The listing builds one solid part. Answer for the finished solid, in the listing's coordinates (mm). A direction names the side the tool comes from. Give positions to 0.01 mm unless a question says otherwise; leave off trailing zeros. Order: outer loops, then holes, each group sorted by start corner. A loop starts at its lowest first (then second) coordinate and runs counter-clockwise, first axis right, second up. Notation, with made-up numbers: (82.25, 22.25) -> (127.25, 22.25) arc R22 cw to (127.25, 39.25) -> close; hole circle Ø9 at (3, 20.5). An arc over 180 degrees is marked (long way). One line per question, with ' | ' between items. Start each with the question number.
```python
from build123d import *

# Parameters (mm, degrees)
SKETCH_2_W          = 2
SKETCH_2_H          = 4.593987872
SKETCH_2_H_2        = 6.667892238
CUT_EXTRUDE_1_DEPTH = 39.5


with BuildPart() as part:
    # 草图1 → 旋转1 (revolve)
    with BuildSketch(Plane.XY, mode=Mode.PRIVATE) as revolve_1_sk:
        Polygon((-23.5, 11), (-26, 11), (-26, 7), (-25.5, 7), (-25.5, 6), (-28, 6), (-28, 5), (-25.5, 5), (-25.5, 4), (-26, 4), (-26, 0), (-23.5, 0), align=None)
    revolve(revolve_1_sk.sketch.rotate(Axis((0, 22.677499451, 0), (0, -1, 0)), 270), axis=Axis((0, 22.677499451, 0), (0, -1, 0)))  # turned: the seam where the file's is

    # 草图2 → 切除-拉伸1 (cut, symmetric)
    with BuildSketch(Plane(origin=(0, 0, 0), x_dir=(0, 0, -1), z_dir=(1, 0, 0))):
        with Locations((0, 11.296993936)):
            Rectangle(SKETCH_2_W, SKETCH_2_H)
        with Locations((0, -1.333946119)):
            Rectangle(SKETCH_2_W, SKETCH_2_H_2)
    extrude(amount=CUT_EXTRUDE_1_DEPTH, both=True, mode=Mode.SUBTRACT)


solid = part.part
```
(1) Determine the mould class of faces 5 (the face through (24.9, 4.5, -5.5)), 6 (the face through (-6, 5, 25)), 7 (the face through (-25, 2, 0)) for opening direction Z: pulls with the +Z half, pulls with the -Z half, needs draft (parallel to the pull), parting line crosses it, or undercut.
(2) The part is cut by section B-B on x = 0. Determine the outline of the cut face in (y, z).
(3) Consider line 1 (Y direction, x = 25.5, z = -4.5); line 2 (X direction, y = 3.5, z = 0); line 3 (Z direction, x = -3.5, y = 6.25). Determine where each line is inside the solid, lowest interval first.
(4) The part is cut by section A-A on z = 0. Determine the outline of the cut face in (x, y).
(5) Given P1, Ø6, axis at y = 9.5, z = -17, coming from the -X side; P2, Ø1.6, axis at x = -25, z = 0, coming from the -Y side; P3, Ø5, axis at y = 9, z = 3.5, coming from the -X side, each flat-ended and moving along its own axis, determine where each tip first touches the part or whether it passes through.
(6) For faces 1 (the face through (15.821, 8.972, -20.633)), 2 (the face through (19.1, 7, 17.2)), 3 (the face through (-25, 10, 1)), 4 (the face through (25, 2, 0)), determine the directions among +Z, -Z, +X, -X, +Y, -Y from which every point of the face is accessible in a straight line to the end or side of a thin tool.
Result sheet:
1) face 5: parting line crosses it | face 6: needs draft | face 7: undercut
2) outline: (0, -26) -> (4, -26) -> (4, -25.5) -> (5, -25.5) -> (5, -28) -> (6, -28) -> (6, -25.5) -> (7, -25.5) -> (7, -26) -> (11, -26) -> (11, -23.5) -> (0, -23.5) -> close; (0, 23.5) -> (11, 23.5) -> (11, 26) -> (7, 26) -> (7, 25.5) -> (6, 25.5) -> (6, 28) -> (5, 28) -> (5, 25.5) -> (4, 25.5) -> (4, 26) -> (0, 26) -> close
3) line 1: y = 0 to 4, 5 to 6, 7 to 11 | line 2: x = -26 to -23.5, 23.5 to 26 | line 3: z = -25.26 to -23.24, 23.24 to 25.26
4) outline: (-28, 5) -> (-25.5, 5) -> (-25.5, 4) -> (-26, 4) -> (-26, 2) -> (-23.5, 2) -> (-23.5, 9) -> (-26, 9) -> (-26, 7) -> (-25.5, 7) -> (-25.5, 6) -> (-28, 6) -> close; (23.5, 2) -> (26, 2) -> (26, 4) -> (25.5, 4) -> (25.5, 5) -> (28, 5) -> (28, 6) -> (25.5, 6) -> (25.5, 7) -> (26, 7) -> (26, 9) -> (23.5, 9) -> close
5) P1: stops at x = -21.91 | P2: stops at y = 2 | P3: stops at x = -25.98
6) face 1: +Y | face 2: none | face 3: +X, -X, +Y | face 4: +X, -X, -Y
